Check sheet for the modelled part. Datum: model origin and axes. Units: mm. A direction names the side the tool comes from. Coordinates: 2 decimals unless noted, no trailing zeros. Order: outer loops, then holes, each group sorted by start corner. A loop starts at its lowest first (then second) coordinate and runs counter-clockwise, first axis right, second up.
1. Draft check along Z on faces 1 (the flat face through (27, 12.743, 63)), 2 (the flat face through (76.2, -193, 57)), 3 (the flat face through (31, -188, 76.2)), 4 (the flat face through (70, -193, 63.5)). Enter one of: released by +Z, released by -Z, zero draft, split by the parting line, or undercut.
2. Set-up check for faces 5 (the flat face through (87, -393.657, 63)), 6 (the flat face through (38.1, -193, 57)), 7 (the flat face through (63.5, -193, 70)), 8 (the flat face through (102.893, -188, 63)), 9 (the flat face through (87, 12.743, 63)): record each of +Z, -Z, +X, -X, +Y, -Y from which the full face is reachable in a straight line by a thin tool's end or side.
3. Thickness scan on line 1 (X direction, y = -161, z = 67.5); line 2 (X direction, y = -373.5, z = 56); line 3 (Y direction, x = 1, z = 46). Record the ranges inside material, lowest first.
4. Gauge pin test, flat ends, axial feed: pin 1 Ø10 at (y, z) = (-244.5, 73) entering from +X; pin 2 Ø4 at (x, z) = (88, 54) entering from +Y; pin 3 Ø14.5 at (x, y) = (-6.65, 18.07) entering from +Z; pin 4 Ø14 at (y, z) = (-114, 57) entering from +X. Record the tip position at first contact, or that the pin passes through.
5. Cross-section at B-B (y = -330). Enter the section's corners in (x, z).
6. Cross-section at A-A (z = 70). Enter the section's corners in (x, y), then the cut area to 3 significant figures.
Autodesk Fusion 360 part; units mm, degrees
sketch "Sketch1" plane through (0, 0, 0) normal (0, 0, 1) x (1, 0, 0)
  line L0 (-20, 30) -> (20.8523, 30)
  line L1 (20.8523, 30) -> (20.8523, -34.8194)
  line L2 (20.8523, -34.8194) -> (-20, -34.8194)
  line L3 (-20, -34.8194) -> (-20, 30)
sketch "Sketch2" plane through (0, 0, 0) normal (0, 0, 1) x (1, 0, 0)
  line L0 (-11.4066, 12.7433) -> (24.3229, 12.7433)
  line L1 (24.3229, 12.7433) -> (24.3229, -393.6567)
  line L2 (24.3229, -393.6567) -> (-11.4066, -393.6567)
  line L3 (-11.4066, -393.6567) -> (-11.4066, 12.7433)
  line L4 (-11.4066, 12.7433) -> (90.1934, 12.7433)
  line L5 (90.1934, 12.7433) -> (90.1934, -393.6567)
  line L6 (90.1934, -393.6567) -> (-11.4066, -393.6567)
  line L7 (-11.4066, -393.6567) -> (-11.4066, 12.7433)
  dimension "d3" = 406.4
  dimension "d4" = 101.6
extrude "Extrude2" add sketch "Sketch2" along normal blind 76.2 contours L1 L4 L5 L6
sketch "Sketch3" plane through (0, -393.6567, 0) normal (0, -1, 0) x (1, 0, 0)
  line L0 (24.3229, 0) -> (90.1934, 0)
  line L1 (90.1934, 0) -> (90.1934, 76.2)
  line L2 (90.1934, 76.2) -> (24.3229, 76.2)
  line L3 (24.3229, 76.2) -> (24.3229, 0)
sketch "Sketch4" plane through (0, -393.6567, 0) normal (0, -1, 0) x (1, 0, 0)
  line L0 (38.1, 63.5) -> (76.2, 63.5)
  line L1 (76.2, 63.5) -> (76.2, 50.8)
  line L2 (76.2, 50.8) -> (38.1, 50.8)
  line L3 (38.1, 50.8) -> (38.1, 63.5)
extrude "Extrude3" cut sketch "Sketch4" against normal blind 444.5
sketch "Sketch5" plane through (0, -393.6567, 0) normal (0, -1, 0) x (1, 0, 0)
  line L0 (50.8, 63.5) -> (63.5, 63.5)
  line L1 (63.5, 63.5) -> (63.5, 76.2)
  line L2 (63.5, 76.2) -> (50.8, 76.2)
  line L3 (50.8, 76.2) -> (50.8, 63.5)
extrude "Extrude4" cut sketch "Sketch5" against normal blind 419.1
sketch "Sketch6" plane through (0, 0, 76.2) normal (0, 0, 1) x (-1, 0, 0)
  line L0 (-50.8, 393.6567) -> (-50.8, -12.7433)
  line L1 (-50.8, -12.7433) -> (-24.3229, -12.7433)
  line L2 (-24.3229, -12.7433) -> (-24.3229, 393.6567)
  line L3 (-24.3229, 393.6567) -> (-50.8, 393.6567)
  line L4 (-6.8471, -24.8983) -> (-111.5412, -24.8983)
  line L5 (-111.5412, -24.8983) -> (-111.5412, 407.05)
  line L6 (-111.5412, 407.05) -> (-6.8471, 407.05)
  line L7 (-6.8471, 407.05) -> (-6.8471, -24.8983)
  circle A0 centre (-15.24, -17.78) radius 5.08
  circle A1 centre (-101.6, -17.78) radius 5.08
  circle A2 centre (-101.6, 398.78) radius 5.08
  circle A3 centre (-17.78, 398.78) radius 5.08
  point P0 (-12.7, 391.3931)
  dimension "d11" = 10.16
  dimension "d12" = 10.16
sketch "Sketch7" plane through (0, 0, 88.9) normal (0, 0, 1) x (-1, 0, 0)
sketch "Sketch8" plane through (0, 0, 0) normal (0, 0, -1) x (1, 0, 0)
  line L0 (24.3229, 393.6567) -> (24.3229, -12.7433)
  line L1 (24.3229, -12.7433) -> (90.1934, -12.7433)
  line L2 (90.1934, -12.7433) -> (90.1934, 393.6567)
  line L3 (90.1934, 393.6567) -> (24.3229, 393.6567)
  line L4 (129.5849, -37.1422) -> (-28.8884, -37.1422)
  line L5 (-28.8884, -37.1422) -> (-28.8884, 441.5791)
  line L6 (-28.8884, 441.5791) -> (129.5849, 441.5791)
  line L7 (129.5849, 441.5791) -> (129.5849, -37.1422)
  circle A0 centre (110.117, -19.8168) radius 6.35
  circle A1 centre (-6.6494, -18.0653) radius 6.35
  circle A2 centre (101.6, 419.1) radius 6.35
  circle A3 centre (0.9404, 412.8027) radius 6.35
  dimension "d15" = 12.7
  dimension "d16" = 12.7
  dimension "d17" = 12.7
  dimension "d18" = 12.7
extrude "Extrude6" add sketch "Sketch8" against normal blind 25.4
sketch "Sketch9" plane through (0, 0, 50.8) normal (0, 0, 1) x (-1, 0, 0)
  line L0 (-76.2, -12.7433) -> (-38.1, -12.7433)
  line L1 (-38.1, -12.7433) -> (-38.1, 393.6567)
  line L2 (-38.1, 393.6567) -> (-76.2, 393.6567)
  line L3 (-76.2, 393.6567) -> (-76.2, -12.7433)
extrude "Extrude7" add 1 faces at (14.3299, -123.04, 25.4) along direction (0, 0, 1) blind 25.4
sketch "Sketch10" plane through (0, -393.6567, 0) normal (0, -1, 0) x (1, 0, 0)
sketch "Sketch11" plane through (0, 37.1422, 0) normal (0, 1, 0) x (-1, 0, 0)
  line L0 (-129.5849, 0) -> (28.8884, 0)
  line L1 (28.8884, 0) -> (28.8884, 50.8)
  line L2 (28.8884, 50.8) -> (-129.5849, 50.8)
  line L3 (-129.5849, 50.8) -> (-129.5849, 0)
extrude "Extrude8" cut 1 faces at (35.4568, -126.9866, 0) along direction (0, 0, 1) blind 38.1
extrude "Extrude9" add 1 faces at (24.3229, -122.7234, 59.2667) along direction (-1, 0, 0) blind 12.7
extrude "Extrude10" add 1 faces at (90.1934, -122.7234, 59.2667) along direction (1, 0, 0) blind 12.7
Data:
1. face 1: zero draft
1. face 2: undercut
1. face 3: released by +Z
1. face 4: undercut
2. face 5: +Z, +X, -X, -Y
2. face 6: +Y, -Y
2. face 7: +Z, +Y, -Y
2. face 8: +Z, +X, +Y, -Y
2. face 9: +Z, +X, -X, +Y
3. line 1: x = 11.62 to 50.8, 63.5 to 102.89
3. line 2: x = 11.62 to 38.1, 76.2 to 102.89
3. line 3: y = -441.58 to -419.15, -406.45 to 37.14
4. pin 1: stops at x = 102.89
4. pin 2: stops at y = 12.74
4. pin 3: stops at z = 50.8
4. pin 4: stops at x = 129.58
5. outline: (-28.89, 38.1) - (129.58, 38.1) - (129.58, 50.8) - (102.89, 50.8) - (102.89, 76.2) - (63.5, 76.2) - (63.5, 63.5) - (76.2, 63.5) - (76.2, 50.8) - (38.1, 50.8) - (38.1, 63.5) - (50.8, 63.5) - (50.8, 76.2) - (11.62, 76.2) - (11.62, 50.8) - (-28.89, 50.8) - close
6. outline: (11.62, -393.66) - (50.8, -393.66) - (50.8, 12.74) - (11.62, 12.74) - close; (63.5, -393.66) - (102.89, -393.66) - (102.89, 12.74) - (63.5, 12.74) - close
6. area: 31,900 mm2
